CAD build for the part. Positions are in the model's coordinates, mm. Round coordinates to 2 decimals unless told otherwise and drop trailing zeros. Order: outer loops, then holes, each group sorted by start corner. A loop starts at its lowest first (then second) coordinate and runs counter-clockwise, first axis right, second up. Notation, with made-up numbers: (11, 61.5) -> (51, 61.5) arc R21 ccw to (51, 70.5) -> close; hole circle Ø10 at (75.25, -13.75). An arc over 180 degrees is marked (long way). Answer as CSV lines item,"result". Start each with the question number.
from build123d import *

# Parameters (mm, degrees)
BOSS_EXTRUDE1_DEPTH = 6
SKETCH2_R           = 2.75
CUT_EXTRUDE1_DEPTH  = 10


with BuildPart() as part:
    # Sketch1 → Boss-Extrude1 (new body)
    with BuildSketch(Plane.XY):
        Polygon((95.814780717, -438.587306273), (95.814780717, -390.58730627), (118.814780717, -390.58730627), (118.814780717, 49.41269373), (95.814780717, 49.41269373), (95.814780717, 97.41269373), (-88.185219283, 97.41269373), (-88.185219283, 49.41269373), (-111.185219283, 49.41269373), (-111.185219283, -390.58730627), (-88.185219283, -390.58730627), (-88.185219283, -438.587306273), (-51.185219283, -438.587306273), (-51.185219283, -415.587306273), (-25.185219283, -415.587306273), (-25.185219283, -438.587306273), align=None)
    extrude(amount=BOSS_EXTRUDE1_DEPTH)

    # Sketch2 → Cut-Extrude1 (cut)
    with BuildSketch(Plane(origin=(0, 0, 0), x_dir=(-1, 0, 0), z_dir=(0, 0, -1))):
        with Locations((-108.814780717, -170.58730627)):
            Circle(SKETCH2_R)
        with Locations((-108.814780717, 4.834891165)):
            Circle(SKETCH2_R)
        with Locations((-108.814780717, -355.336655309)):
            Circle(SKETCH2_R)
        with Locations((101.185219283, 4.834891165)):
            Circle(SKETCH2_R)
        with Locations((101.185219283, -170.58730627)):
            Circle(SKETCH2_R)
        with Locations((101.185219283, -355.336655309)):
            Circle(SKETCH2_R)
    extrude(amount=-CUT_EXTRUDE1_DEPTH, mode=Mode.SUBTRACT)


solid = part.part
Item 1: Pin check, flat tips, straight feed: pin 1 (1.8 mm diameter, centred on x = 113, z = 3.5, fed in from +Y); pin 2 (1.8 mm diameter, centred on y = -423, z = 2.5, fed in from +X); pin 3 (9 mm diameter, centred on x = 108.81, y = 4.83, fed in from -Z); pin 4 (3 mm diameter, centred on x = -94, z = 4.5, fed in from -Y). Stop position of each tip, or through.
Item 2: Probe line 1 (Y direction, x = 109.5, z = 2); line 2 (Y direction, x = -100, z = 5.15); line 3 (X direction, y = 5.5, z = 3.85). List the from-to ranges inside material, lowest first.
Item 3: Band-saw the part on B-B, the plane x = -33.5. Give the cut face in (y, z).
Item 4: Band-saw the part on A-A, the plane z = 4.5. Give the cut face in (x, y), and give its area (3 significant figures).
Values:
1,pin 1,"y = 49.41"
1,pin 2,"x = 95.81"
1,pin 3,"z = 0"
1,pin 4,"y = -390.59"
2,line 1,"-390.59 to -358, -352.67 to -173.25, -167.92 to 2.17, 7.5 to 49.41"
2,line 2,"-390.59 to -357.82, -352.86 to -173.07, -168.11 to 2.35, 7.32 to 49.41"
2,line 3,"-111.19 to -103.85, -98.52 to 106.15, 111.48 to 118.81"
3,outline,"(-415.59, 0) -> (97.41, 0) -> (97.41, 6) -> (-415.59, 6) -> close"
4,outline,"(-111.19, -390.59) -> (-88.19, -390.59) -> (-88.19, -438.59) -> (-51.19, -438.59) -> (-51.19, -415.59) -> (-25.19, -415.59) -> (-25.19, -438.59) -> (95.81, -438.59) -> (95.81, -390.59) -> (118.81, -390.59) -> (118.81, 49.41) -> (95.81, 49.41) -> (95.81, 97.41) -> (-88.19, 97.41) -> (-88.19, 49.41) -> (-111.19, 49.41) -> close; hole circle Ø5.5 at (-101.19, -355.34); hole circle Ø5.5 at (-101.19, -170.59); hole circle Ø5.5 at (-101.19, 4.83); hole circle Ø5.5 at (108.81, -355.34); hole circle Ø5.5 at (108.81, -170.59); hole circle Ø5.5 at (108.81, 4.83)"
4,area,"118,000 mm²"
